```python
from build123d import *

# Parameters (mm, degrees)
F0_R      = 7.1
F1_DEPTH  = 9
F2_R      = 0.75
F3_DEPTH  = 5
F4_R      = 1
F5_DEPTH  = 3
F6_R      = 2.75
F7_DEPTH  = 3
F8_R      = 0.7
F9_DEPTH  = 0.75
F10_R     = 2
F11_DEPTH = 0.3
F12_R     = 0.8227174872
F13_DEPTH = 1
F14_SIZE  = 0.8


with BuildPart() as f1:
    # F0 (on Top) → F1 (new body)
    with BuildSketch(Plane.XY):
        Circle(F0_R)
    extrude(amount=F1_DEPTH)

    # F2 (on face) → F3 (join)
    with BuildSketch(Plane.XY.offset(9)):
        Circle(F2_R)
    extrude(amount=F3_DEPTH)

    # F4 (on face) → F5 (cut)
    with BuildSketch(Plane.XY.offset(9)):
        with Locations((3.1819805153, 3.1819805153)):
            Circle(F4_R)
        with Locations((-3.1819805153, 3.1819805153)):
            Circle(F4_R)
        with Locations((-3.1819805153, -3.1819805153)):
            Circle(F4_R)
        with Locations((3.1819805153, -3.1819805153)):
            Circle(F4_R)
    extrude(amount=-F5_DEPTH, mode=Mode.SUBTRACT)

    # F6 (on face) → F7 (join)
    with BuildSketch(Plane(origin=(0, 0, 0), x_dir=(1, 0, 0), z_dir=(0, 0, -1))):
        Circle(F6_R)
    extrude(amount=F7_DEPTH)

    # F8 (on face) → F9 (join, symmetric)
    with BuildSketch(Plane(origin=(0, 0, -3), x_dir=(1, 0, 0), z_dir=(0, 0, -1))):
        with BuildLine():
            ThreePointArc((4.185713319, -1.25), (5.450081641, 0), (4.185713319, 1.25))
            ThreePointArc((4.185713319, 1.25), (3.0570558213, 1.4644635871), (2.1, 2.1))
            ThreePointArc((2.1, 2.1), (1.4644635871, 3.0570558213), (1.25, 4.185713319))
            ThreePointArc((1.25, 4.185713319), (0, 5.450081641), (-1.25, 4.185713319))
            ThreePointArc((-1.25, 4.185713319), (-1.4644635871, 3.0570558213), (-2.1, 2.1))
            ThreePointArc((-2.1, 2.1), (-3.0570558213, 1.4644635871), (-4.185713319, 1.25))
            ThreePointArc((-4.185713319, 1.25), (-5.450081641, 0), (-4.185713319, -1.25))
            ThreePointArc((-4.185713319, -1.25), (-3.0570558213, -1.4644635871), (-2.1, -2.1))
            ThreePointArc((-2.1, -2.1), (-1.4644635871, -3.0570558213), (-1.25, -4.185713319))
            ThreePointArc((-1.25, -4.185713319), (0, -5.450081641), (1.25, -4.185713319))
            ThreePointArc((1.25, -4.185713319), (1.4644635871, -3.0570558213), (2.1, -2.1))
            ThreePointArc((2.1, -2.1), (3.0570558213, -1.4644635871), (4.185713319, -1.25))
        make_face()
        with Locations((0, -4.2)):
            Circle(F8_R, mode=Mode.SUBTRACT)
        with Locations((-4.2, 0)):
            Circle(F8_R, mode=Mode.SUBTRACT)
        with Locations((4.2, 0)):
            Circle(F8_R, mode=Mode.SUBTRACT)
        with Locations((0, 4.2)):
            Circle(F8_R, mode=Mode.SUBTRACT)
    extrude(amount=F9_DEPTH, both=True)

    # F10 (on face) → F11 (join)
    with BuildSketch(Plane(origin=(0, 0, -3.75), x_dir=(1, 0, 0), z_dir=(0, 0, -1))):
        Circle(F10_R)
    extrude(amount=F11_DEPTH)

    # F12 (on face) → F13 (join)
    with BuildSketch(Plane(origin=(0, 0, -4.05), x_dir=(1, 0, 0), z_dir=(0, 0, -1))):
        Circle(F12_R)
    extrude(amount=F13_DEPTH)

    # F14
    f14_edges = [f1.edges().sort_by_distance(p)[0] for p in [
        (-7.1, 0, 9),
    ]]
    chamfer(f14_edges, length=F14_SIZE)


solid = f1.part
```
CAD build for the part. Positions are in the model's coordinates, mm. A direction names the side the tool comes from. Coordinates: 2 decimals unless noted, no trailing zeros. Write each loop counter-clockwise with the first axis right and the second up, starting at its lowest first coordinate (ties: lowest second). Pieces come first, ordered by that corner, then holes.
(1) Drill centre lines: probe 1 along Z at (x, y) = (0.5, 5.25); probe 2 along Y at (x, z) = (-4.2, -3.15); probe 3 along X at (y, z) = (-3.5, 7.5). Where is each one in solid material? Low to high.
(2) Cut at C-C, the plane z = 6.5. List the corners of the cut face in (x, y).
(3) 3-axis set-ups, long thin cutter, end or side, ignore diameter. For faces 1 (the face through (-0.92, 7.04, 4.04)), 2 (the face through (-3, 3, 6)), 3 (the face through (-3.532, -0.21, -2.99)), 4 (the face through (0, 3, -2.25)): which of +Z, -Z, +X, -X, +Y, -Y reach the whole face in a straight line?
(4) Two-plate mould, pull along X, no slides. Class faces 5 (the face through (0, 0, 14)), 6 (the face through (4.136, -2.882, 7.521)), 7 (the face through (0.03, -5.45, -3.01)): +X half, -X half, draft (parallel to the pull), parting line (faces both ways), or undercut.
(5) Flat gauge pins, fed straight in: pin 1 (1.5 mm diameter, centred on y = -4, z = 8, fed in from -X); pin 2 (2.5 mm diameter, centred on x = -3.18, y = -3.18, fed in from +Z); pin 3 (5 mm diameter, centred on x = -4.5, z = 1.5, fed in from +Y). Where does each tip first touch, or does it go through?
(6) Cut at D-D, the plane z = 10.25. List the corners of the cut face in (x, y), and give its area (3 significant figures).
(7) Cut at A-A, the plane x = 0. Count the separate pieces of the cut face and the enclosed holes in it, and give its area (3 significant figures).
(8) Cut at B-B, the plane z = -2.5. List the corners of the cut face in (x, y), and give its area (3 significant figures).
Geometry says:
1. probe 1: z = -3.75 to -2.25, 0 to 9
1. probe 2: y = -1.25 to -0.7, 0.7 to 1.25
1. probe 3: x = -6.18 to -4.13, -2.23 to 2.23, 4.13 to 6.18
2. outline: circle Ø14.2 at (0, 0); hole circle Ø2 at (-3.18, -3.18); hole circle Ø2 at (-3.18, 3.18); hole circle Ø2 at (3.18, -3.18); hole circle Ø2 at (3.18, 3.18)
3. face 1: +Z, -Z
3. face 2: +Z
3. face 3: -Z
3. face 4: none
4. face 5: draft
4. face 6: undercut
4. face 7: parting line
5. pin 1: stops at x = -6.31
5. pin 2: stops at z = 9
5. pin 3: stops at y = 6.81
6. outline: circle Ø1.5 at (0, 0)
6. area: 1.77 mm2
7. separate pieces: 3
7. enclosed holes: 0
7. area: 162 mm2
8. outline: (-4.19, -1.25) arc R2.9 cw to (-1.25, -4.19) arc R1.25 ccw (long way) to (1.25, -4.19) arc R2.9 cw to (4.19, -1.25) arc R1.25 ccw (long way) to (4.19, 1.25) arc R2.9 cw to (1.25, 4.19) arc R1.25 ccw (long way) to (-1.25, 4.19) arc R2.9 cw to (-4.19, 1.25) arc R1.25 ccw (long way) to start; hole circle Ø1.4 at (-4.2, 0); hole circle Ø1.4 at (0, -4.2); hole circle Ø1.4 at (0, 4.2); hole circle Ø1.4 at (4.2, 0)
8. area: 46.6 mm2
